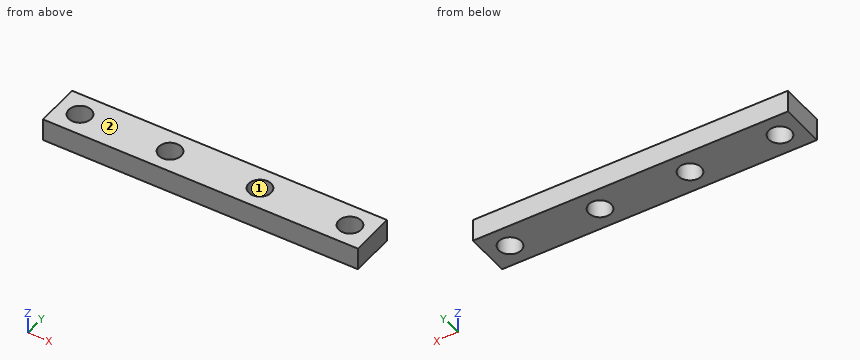
```python
from build123d import *

# Parameters (mm, degrees)
SKETCH2_W           = 44.45
SKETCH2_H           = 6.35
BOSS_EXTRUDE1_DEPTH = 3.175
SKETCH3_R           = 1.5875
CUT_EXTRUDE1_DEPTH  = 4.175


with BuildPart() as part:
    # Sketch2 → Boss-Extrude1 (new body)
    with BuildSketch(Plane.XY):
        Rectangle(SKETCH2_W, SKETCH2_H)
    extrude(amount=BOSS_EXTRUDE1_DEPTH)

    # Sketch3 → Cut-Extrude1 (cut, through all)
    with BuildSketch(Plane.XY.offset(3.175)):
        with Locations((-6.35, 0)):
            Circle(SKETCH3_R)
        with Locations((-19.05, 0)):
            Circle(SKETCH3_R)
    cut_extrude1 = extrude(amount=-CUT_EXTRUDE1_DEPTH, mode=Mode.SUBTRACT)

    # Mirror1: Cut-Extrude1 across plane
    add(cut_extrude1.mirror(Plane(origin=(0, 0, 0), x_dir=(0, 0, 1), z_dir=(1, 0, 0))), mode=Mode.SUBTRACT)


solid = part.part
```
For this review, take the finished solid that the model builds, in its own axes (mm). Face numbers are marked on the shaded views. Round coordinates to 2 decimals unless told otherwise and drop trailing zeros. Loops run counter-clockwise (first coordinate to the right, second up) from the corner with the lowest first, then second, coordinate; pieces in that order, holes last.
Q1. Insertion check: pin 1 Ø2.5 at (x, y) = (19.05, 0) entering from -Z. The pin has a flat end and moves straight along its axis. Give the tip position at first contact, or say it passes through.
Result sheet:
pin 1: passes through
Q2. Add section C-C on z = 2.1. Give the number of separate pieces and of enclosed holes in the cut face, plus the area to 3 significant figures.
Result sheet:
separate pieces: 1
enclosed holes: 4
area: 251 mm2
Q3. Mouldability with a two-part tool opening along X and no side actions: class the marked faces 1 and 2 as +X half, -X half, draft (parallel to the pull), parting line (faces both ways), or undercut.
Result sheet:
face 1: undercut
face 2: draft
Q4. To check wall thickness, follow line 1 along Y through (x, z) = (6.35, 2.2) (1 decimal); line 2 along X through (y, z) = (-0.75, 3) (3 decimals); line 3 along X through (y, z) = (1, 0.45) (3 decimals). State the ranges of each line that lie inside material, in increasing order.
Result sheet:
line 1: y = -3.2 to -1.6, 1.6 to 3.2
line 2: x = -22.225 to -20.449, -17.651 to -7.749, -4.951 to 4.951, 7.749 to 17.651, 20.449 to 22.225
line 3: x = -22.225 to -20.283, -17.817 to -7.583, -5.117 to 5.117, 7.583 to 17.817, 20.283 to 22.225
Q5. Add section B-B on x = -6.35. Write out the cut boundary in (y, z) (1 decimal), plus the area to 3 significant figures.
Result sheet:
outline: (-3.2, 0) - (-1.6, 0) - (-1.6, 3.2) - (-3.2, 3.2) - close; (1.6, 0) - (3.2, 0) - (3.2, 3.2) - (1.6, 3.2) - close
area: 10.1 mm2
Q6. Add section A-A on y = 0. Write out the cut boundary in (x, z) (1 decimal), plus the area to 3 significant figures.
Result sheet:
outline: (-22.2, 0) - (-20.6, 0) - (-20.6, 3.2) - (-22.2, 3.2) - close; (-17.5, 0) - (-7.9, 0) - (-7.9, 3.2) - (-17.5, 3.2) - close; (-4.8, 0) - (4.8, 0) - (4.8, 3.2) - (-4.8, 3.2) - close; (7.9, 0) - (17.5, 0) - (17.5, 3.2) - (7.9, 3.2) - close; (20.6, 0) - (22.2, 0) - (22.2, 3.2) - (20.6, 3.2) - close
area: 101 mm2
